Geometry check sheet. Reference: the model listing, model coordinates, mm. Coordinates: 2 decimals unless noted, no trailing zeros. Order: outer loops, then holes, each group sorted by start corner. A loop starts at its lowest first (then second) coordinate and runs counter-clockwise, first axis right, second up. Notation, with made-up numbers: (82.25, 72) -> (129.25, 72) arc R23 ccw to (129.25, 88) -> close; hole circle Ø9 at (74, 76). An arc over 180 degrees is marked (long way). Answer in a Markdown table with one row per item. Add a question column.
```python
from build123d import *

# Parameters (mm, degrees)
F0_R     = 8
F1_DEPTH = 5
F2_R     = 5
F3_R     = 2
F5_SIZE  = 0.6


with BuildPart() as f1:
    # F0 (on Front) → F1 (new body)
    with BuildSketch(Plane.XZ):
        with BuildLine():
            ThreePointArc((-59.542741, 24.134741), (-52.111337, 9.81657), (-39.6, 20))
            ThreePointArc((-39.6, 20), (-47.888663, 30.18343), (-59.542741, 24.134741))
        make_face()
        with Locations((-50, 20)):
            Circle(F0_R, mode=Mode.SUBTRACT)
        with BuildLine():
            Line((0, 20), (-39.6, 20))
            ThreePointArc((-39.6, 20), (-52.111337, 9.81657), (-59.542741, 24.134741))
            Line((-59.542741, 24.134741), (-70, 0))
            Line((-70, 0), (-30, 0))
            Line((-30, 0), (0, 0))
            Line((0, 0), (0, 20))
        make_face()
    extrude(amount=F1_DEPTH)

    # F2
    f2_edges = [f1.edges().sort_by_distance(p)[0] for p in [
        (-39.6, -2.5, 20),
        (-59.542741, -2.5, 24.134741),
    ]]
    fillet(f2_edges, radius=F2_R)

    # F3
    f3_edges = [f1.edges().sort_by_distance(p)[0] for p in [
        (-70, -2.5, 0),
    ]]
    fillet(f3_edges, radius=F3_R)

    # F4: F1 across face


with BuildPart() as f1_1:
    add(f1.part)
    add(f1.part.mirror(Plane(origin=(0, -2.5, 10), x_dir=(0, 1, 0), z_dir=(1, 0, 0))))

    # F5
    f5_edges = [f1_1.edges().sort_by_distance(p)[0] for p in [
        (-64.165822, -5, 13.464942),
        (-68.625628, -5, 0.90234),
        (0, -5, 0),
        (68.625628, -5, 0.90234),
        (64.165822, -5, 13.464942),
        (49.593464, -5, 30.392051),
        (38.339723, -5, 20.930793),
        (0, -5, 20),
        (-38.339723, -5, 20.930793),
        (-49.593464, -5, 30.392051),
        (-58, -5, 20),
        (58, -5, 20),
        (-64.165822, 0, 13.464942),
        (-68.625628, 0, 0.90234),
        (0, 0, 0),
        (68.625628, 0, 0.90234),
        (64.165822, 0, 13.464942),
        (49.593464, 0, 30.392051),
        (38.339723, 0, 20.930793),
        (0, 0, 20),
        (-38.339723, 0, 20.930793),
        (-49.593464, 0, 30.392051),
        (-58, 0, 20),
        (58, 0, 20),
    ]]
    chamfer(f5_edges, length=F5_SIZE)


solid = f1_1.part
```
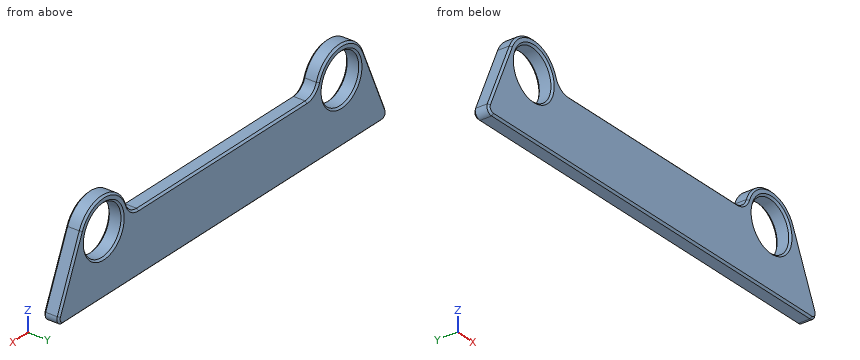
(1) Cross-section at A-A (x = 50). Enter the section's corners in (y, z).
(2) Go/stop test with flat-tipped pins: P1, Ø14.5, axis at x = 50, z = 20, coming from the -Y side; P2, Ø3, axis at x = 33.5, y = -2, coming from the +Z side. Record where each tip stops, or that it passes through.
(3) Cross-section at D-D (z = 21.5). Give the number of separate pieces and of enclosed holes in the cut face, plus the area to 3 significant figures.
(4) Cross-section at B-B (y = -3.1). Enter the section's corners in (x, z).
(5) Cross-section at C-C (x = 6.5). Enter the section's corners in (y, z).
(6) Scan lines: line 1 along Z through (x, y) = (50, -2.35); line 2 along X through (y, z) = (-1.6, 20.5); line 3 along X through (y, z) = (-3.5, 22). Record each from-to range of solid material in increasing order.
Checks:
| question | item | result |
|---|---|---|
| 1 | outline | (-5, 0.6) -> (-4.4, 0) -> (-0.6, 0) -> (0, 0.6) -> (0, 11.4) -> (-0.6, 12) -> (-4.4, 12) -> (-5, 11.4) -> close; (-5, 28.6) -> (-4.4, 28) -> (-0.6, 28) -> (0, 28.6) -> (0, 29.8) -> (-0.6, 30.4) -> (-4.4, 30.4) -> (-5, 29.8) -> close |
| 2 | P1 | through |
| 2 | P2 | z = 20 |
| 3 | separate pieces | 4 |
| 3 | enclosed holes | 0 |
| 3 | area | 56.4 mm² |
| 4 | outline | (-68.79, 2.8) arc R2 ccw to (-66.95, 0) -> (66.95, 0) arc R2 ccw to (68.79, 2.8) -> (59.54, 24.13) arc R10.4 ccw to (40.16, 23.38) arc R5 cw to (35.43, 20) -> (-35.43, 20) arc R5 cw to (-40.16, 23.38) arc R10.4 ccw to (-59.54, 24.13) -> close; hole circle Ø16 at (-50, 20); hole circle Ø16 at (50, 20) |
| 5 | outline | (-5, 0.6) -> (-4.4, 0) -> (-0.6, 0) -> (0, 0.6) -> (0, 19.4) -> (-0.6, 20) -> (-4.4, 20) -> (-5, 19.4) -> close |
| 6 | line 1 | 0 to 12, 28 to 30.4 |
| 6 | line 2 | -61.12 to -57.98, -42.02 to -37.61, 37.61 to 42.02, 57.98 to 61.12 |
| 6 | line 3 | -60.47 to -57.75, -42.25 to -39.43, 39.43 to 42.25, 57.75 to 60.47 |
